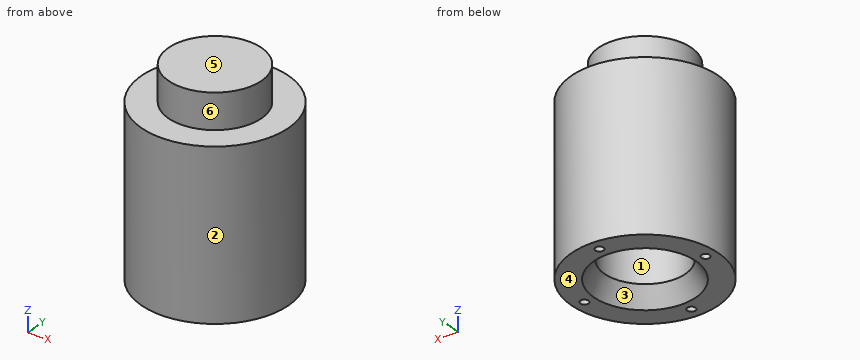
from build123d import *

# Parameters (mm, degrees)
F_4_40_TAPPED_HOLE1_D     = 2.2606
F_4_40_TAPPED_HOLE1_DEPTH = 9.525
F_4_40_TAPPED_HOLE1_TIP   = 0.679152758


with BuildPart() as part:
    # Sketch1 → Revolve1 (revolve)
    with BuildSketch(Plane(origin=(0, 0, 0), x_dir=(0, 0, -1), z_dir=(1, 0, 0))):
        Polygon((0, 0), (0, 12.6492), (9.525, 12.6492), (9.525, 20), (54.525, 20), (54.525, 13.886751346), (49.525, 11), (19.525, 11), (19.525, 0), align=None)
    revolve(axis=Axis((0, 0, -19.525), (0, 0, 1)))

    # #4-40 Tapped Hole1
    with Locations(Plane(origin=(0, 0, -54.525), x_dir=(-1, 0, 0), z_dir=(0, 0, -1))):
        with Locations((16.8275, 0), (0.223849371, 16.826011046), (0, -16.8275), (-16.8275, 0)):
            Hole(F_4_40_TAPPED_HOLE1_D / 2, depth=F_4_40_TAPPED_HOLE1_DEPTH)
            with Locations((0, 0, -(F_4_40_TAPPED_HOLE1_DEPTH + F_4_40_TAPPED_HOLE1_TIP / 2))):  # 118° drill point
                Cone(0, F_4_40_TAPPED_HOLE1_D / 2, F_4_40_TAPPED_HOLE1_TIP, mode=Mode.SUBTRACT)


solid = part.part
Here's how the part is built. I have some questions about the finished solid (model axes, mm). Face numbers are marked on the shaded views. A direction names the side the tool comes from. Coordinates: 2 decimals unless noted, no trailing zeros. Loops run counter-clockwise (first coordinate to the right, second up) from the corner with the lowest first, then second, coordinate; pieces in that order, holes last.
1. Imagine slicing it at B-B, the plane z = -7. Please give me the cut outline in (x, y), and give its area (3 significant figures).
2. For P1, Ø1.4, axis at x = -16.83, y = 0, coming from the -Z side; P2, Ø1, axis at x = -12.5, z = -41, coming from the -Y side; P3, Ø1.5, axis at x = -12, z = -20, coming from the -Y side, each with a flat end and sliding along its axis, tell me the tip position at first contact or that it passes through.
3. Imagine slicing it at C-C, the plane y = -15. Please give me the cut outline in (x, z) (3 decimals), and give its area (3 significant figures).
4. Imagine slicing it at D-D, the plane z = -16.5. Please give me the cut outline in (x, y).
5. I need wall thicknesses on L1, parallel to Y at x = 0, z = -35; L2, parallel to Y at x = 0, z = -48. Which ranges of each line are inside material? Lowest first, please.
6. Imagine slicing it at A-A, the plane z = -27.5. Please give me the cut outline in (x, y), and give its area (3 significant figures).
7. For the marked faces 5 and 6, which set-ups out of +Z, -Z, +X, -X, +Y, -Y let a thin tool reach every point of the face, with its end or its side?
8. If we mould it in two halves opening along X, with no side actions, what happens to the marked faces 1, 2, 3 and 4? For each: pulls with the +X half, pulls with the -X half, needs draft (parallel to the pull), parting line crosses it, or undercut.
Taken from the geometry:
1. outline: circle Ø25.3 at (0, 0)
1. area: 503 mm2
2. P1: stops at z = -44.74
2. P2: stops at y = -16
2. P3: stops at y = -16.54
3. outline: (-13.229, -54.525) - (13.229, -54.525) - (13.229, -9.525) - (-13.229, -9.525) - close
3. area: 1,190 mm2
4. outline: circle Ø40 at (0, 0)
5. L1: y = -20 to -11, 11 to 20
5. L2: y = -20 to -17.96, -15.7 to -11, 11 to 15.72, 17.93 to 20
6. outline: circle Ø40 at (0, 0); hole circle Ø22 at (0, 0)
6. area: 877 mm2
7. face 5: +Z, +X, -X, +Y, -Y
7. face 6: +Z
8. face 1: undercut
8. face 2: parting line crosses it
8. face 3: undercut
8. face 4: needs draft
